from build123d import *

# Parameters (mm, degrees)
F0_R     = 12.7
F1_DEPTH = 28.448
F2_R     = 2.54
F3_R     = 152.4
F3_R_2   = 127
F4_DEPTH = 1.524


with BuildPart() as f1:
    # F0 (on Front) → F1 (new body)
    with BuildSketch(Plane.XZ):
        with BuildLine():
            ThreePointArc((0, 203.2), (-143.684098, -143.684098), (203.2, 0))
            ThreePointArc((203.2, 0), (161.209399, 123.700322), (52.59203, 196.276128))
            Line((52.59203, 196.276128), (50.126779, 187.075684))
            ThreePointArc((50.126779, 187.075684), (56.915364, 182.539697), (59.539777, 174.808426))
            ThreePointArc((59.539777, 174.808426), (54.571047, 164.732839), (43.552775, 162.541168))
            Line((43.552775, 162.541168), (0, 0))
            Line((0, 0), (0, 203.2))
        make_face()
        with Locations((-127.96865, -127.96865)):
            Circle(F0_R, mode=Mode.SUBTRACT)
        with Locations((-46.839777, -174.808426)):
            Circle(F0_R, mode=Mode.SUBTRACT)
        with Locations((-174.808426, -46.839777)):
            Circle(F0_R, mode=Mode.SUBTRACT)
        with Locations((46.839777, -174.808426)):
            Circle(F0_R, mode=Mode.SUBTRACT)
        with Locations((127.96865, -127.96865)):
            Circle(F0_R, mode=Mode.SUBTRACT)
        with Locations((174.808426, -46.839777)):
            Circle(F0_R, mode=Mode.SUBTRACT)
        with Locations((-174.808426, 46.839777)):
            Circle(F0_R, mode=Mode.SUBTRACT)
        with Locations((-127.96865, 127.96865)):
            Circle(F0_R, mode=Mode.SUBTRACT)
        with Locations((-46.839777, 174.808426)):
            Circle(F0_R, mode=Mode.SUBTRACT)
        with Locations((174.808426, 46.839777)):
            Circle(F0_R, mode=Mode.SUBTRACT)
        with Locations((127.96865, 127.96865)):
            Circle(F0_R, mode=Mode.SUBTRACT)
        with BuildLine():
            Line((50.126779, 187.075684), (52.59203, 196.276128))
            ThreePointArc((52.59203, 196.276128), (26.522922, 201.461596), (0, 203.2))
            Line((0, 203.2), (0, 0))
            Line((0, 0), (43.552775, 162.541168))
            ThreePointArc((43.552775, 162.541168), (34.572519, 178.095428), (50.126779, 187.075684))
        make_face()
    extrude(amount=F1_DEPTH)

    # F2
    f2_edges = [f1.edges().sort_by_distance(p)[0] for p in [
        (-203.2, -28.448, 0),
        (-203.2, 0, 0),
    ]]
    fillet(f2_edges, radius=F2_R)

    # F3 (on face) → F4 (join)
    with BuildSketch(Plane.XZ.offset(28.448)):
        Circle(F3_R)
        Circle(F3_R_2, mode=Mode.SUBTRACT)
    extrude(amount=F4_DEPTH)


solid = f1.part
Verification items for the finished model (mm, model axes). A direction names the side the tool comes from. Give positions to 0.01 mm unless a question says otherwise; leave off trailing zeros. Answer as CSV lines item,"result".
Q1. Sectioned sample at A-A on y = -17.5. Count the separate pieces of the cut face and the enclosed holes in it, plus the area to 3 significant figures.
Solutions:
separate pieces,"1"
enclosed holes,"12"
area,"124,000 mm²"
Q2. Depth check by flat-ended pin: pin 1 (20.5 mm diameter, centred on x = -174.81, z = 46.84, fed in from +Y); pin 2 (3 mm diameter, centred on x = 7.5, y = -5, fed in from +Z); pin 3 (1.5 mm diameter, centred on x = 47, y = -9, fed in from -Z); pin 4 (5 mm diameter, centred on x = -151.5, y = -3, fed in from +Z). Enter the tip coordinate at first touch or a pass-through.
Solutions:
pin 1,"passes through"
pin 2,"stops at z = 203.11"
pin 3,"stops at z = -197.87"
pin 4,"stops at z = 138.16"
Q3. Access from +Z, -Z, +X, -X, +Y, -Y to the whole of each face (thin tool, end or side, straight path). Record for faces 1 (the cylindrical face through (-40.01, -14.02, -164.1)), 2 (the cylindrical face through (-27.53, -29.2, -123.98)).
Solutions:
face 1,"+Y, -Y"
face 2,"-Y"
Q4. Scan lines: probe 1 along X at (y, z) = (-13.25, 166); probe 2 along Z at (x, y) = (125.5, -2.75); probe 3 along Z at (x, y) = (118, -8). Record each from-to range of solid material in increasing order.
Solutions:
probe 1,"x = -117.19 to -55.99, -37.69 to 37.69, 55.99 to 117.19"
probe 2,"z = -159.81 to -140.43, -115.51 to 115.51, 140.43 to 159.81"
probe 3,"z = -165.43 to -135.84, -120.1 to 120.1, 135.84 to 165.43"
Q5. Release check for a two-part mould opening along Z. For faces 3 (the flat face through (-75, -28.448, 135)), 4 (the cylindrical face through (-120.94, -29.2, -92.73)), 5 (the cylindrical face through (134.796, -14.025, 138.677)) record: +Z half, -Z half, draft (parallel to the pull), parting line (faces both ways), or undercut.
Solutions:
face 3,"draft"
face 4,"parting line"
face 5,"undercut"
